Could you check a few things on this model? Use its own coordinates, in mm. Face numbers are marked on the shaded views. A direction names the side the tool comes from. Coordinates: 2 decimals unless noted, no trailing zeros. Loops run counter-clockwise (first coordinate to the right, second up) from the corner with the lowest first, then second, coordinate; pieces in that order, holes last.
from build123d import *

# Parameters (mm, degrees)
SKETCH2_W      = 69
SKETCH2_H      = 24.5
EXTRUDE1_DEPTH = 12.5
SKETCH3_R      = 1.65
EXTRUDE2_DEPTH = 39.685430074
SKETCH4_W      = 3
SKETCH4_H      = 24.5
EXTRUDE3_DEPTH = 5


with BuildPart() as part:
    # Sketch2 → Extrude1 (new body)
    with BuildSketch(Plane.XY):
        Rectangle(SKETCH2_W, SKETCH2_H)
    extrude(amount=EXTRUDE1_DEPTH)

    # Sketch3 → Extrude2 (cut, through all)
    with BuildSketch(Plane.XY.offset(12.5)):
        with Locations((-21.5, 0)):
            Circle(SKETCH3_R)
        with Locations((13.5, 0)):
            Circle(SKETCH3_R)
    extrude(amount=-EXTRUDE2_DEPTH, mode=Mode.SUBTRACT)

    # Sketch4 → Extrude3 (add)
    with BuildSketch(Plane.XY.offset(12.5)):
        with Locations((33, 0)):
            Rectangle(SKETCH4_W, SKETCH4_H)
        with Locations((-5, 0)):
            Rectangle(SKETCH4_W, SKETCH4_H)
    extrude(amount=EXTRUDE3_DEPTH)


solid = part.part
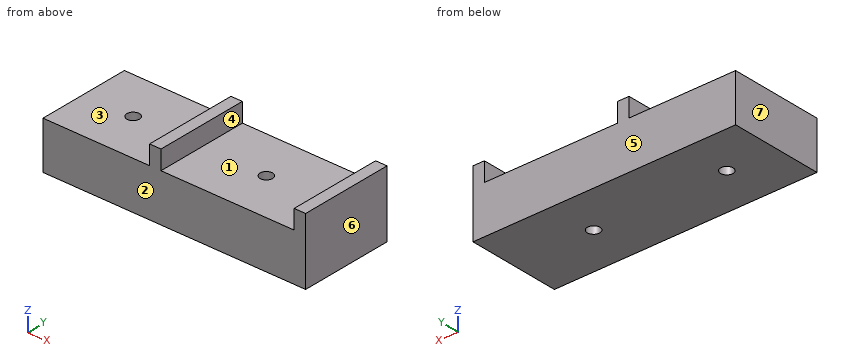
(1) We'd pull the mould along X, two halves only. Please class the marked faces 4, 5, 6 and 7: +X half, -X half, draft (parallel to the pull), parting line (faces both ways), or undercut.
Answers:
face 4: undercut
face 5: draft
face 6: +X half
face 7: -X half
(2) Imagine slicing it at D-D, the plane x = 21. Write out the boundary of the cut face in (y, z), and give its area (3 significant figures).
Answers:
outline: (-12.25, 0) - (12.25, 0) - (12.25, 12.5) - (-12.25, 12.5) - close
area: 306 mm2
(3) I need wall thicknesses on probe 1 along X at (y, z) = (10.5, 14.5); probe 2 along X at (y, z) = (-0.75, 1.5); probe 3 along Y at (x, z) = (13.5, 3). Which ranges of each line are inside material? Lowest first, please.
Answers:
probe 1: x = -6.5 to -3.5, 31.5 to 34.5
probe 2: x = -34.5 to -22.97, -20.03 to 12.03, 14.97 to 34.5
probe 3: y = -12.25 to -1.65, 1.65 to 12.25
(4) Imagine slicing it at A-A, the plane y = 0. Write out the boundary of the cut face in (x, z), and give its area (3 significant figures).
Answers:
outline: (-34.5, 0) - (-23.15, 0) - (-23.15, 12.5) - (-34.5, 12.5) - close; (-19.85, 0) - (11.85, 0) - (11.85, 12.5) - (-3.5, 12.5) - (-3.5, 17.5) - (-6.5, 17.5) - (-6.5, 12.5) - (-19.85, 12.5) - close; (15.15, 0) - (34.5, 0) - (34.5, 17.5) - (31.5, 17.5) - (31.5, 12.5) - (15.15, 12.5) - close
area: 810 mm2
(5) Imagine slicing it at B-B, the plane x = 13.5. Write out the boundary of the cut face in (y, z), and give its area (3 significant figures).
Answers:
outline: (-12.25, 0) - (-1.65, 0) - (-1.65, 12.5) - (-12.25, 12.5) - close; (1.65, 0) - (12.25, 0) - (12.25, 12.5) - (1.65, 12.5) - close
area: 265 mm2
(6) For pin 1 (12 mm diameter, centred on x = 9, y = -5.5, fed in from +Z); pin 2 (1.5 mm diameter, centred on y = -2, z = 15.5, fed in from -X); pin 3 (3 mm diameter, centred on x = 13.5, y = 0, fed in from +Z), each with a flat end and sliding along its axis, tell me the tip position at first contact or that it passes through.
Answers:
pin 1: stops at z = 12.5
pin 2: stops at x = -6.5
pin 3: passes through
(7) Which directions (+Z, -Z, +X, -X, +Y, -Y) give clear straight access to the entire face, cutting with the end or side of a thin tool? Please do the marked faces 1, 2 and 3.
Answers:
face 1: +Z, +Y, -Y
face 2: +Z, -Z, +X, -X, -Y
face 3: +Z, -X, +Y, -Y
(8) Imagine slicing it at C-C, the plane y = 8. Write out the boundary of the cut face in (x, z).
Answers:
outline: (-34.5, 0) - (34.5, 0) - (34.5, 17.5) - (31.5, 17.5) - (31.5, 12.5) - (-3.5, 12.5) - (-3.5, 17.5) - (-6.5, 17.5) - (-6.5, 12.5) - (-34.5, 12.5) - close
